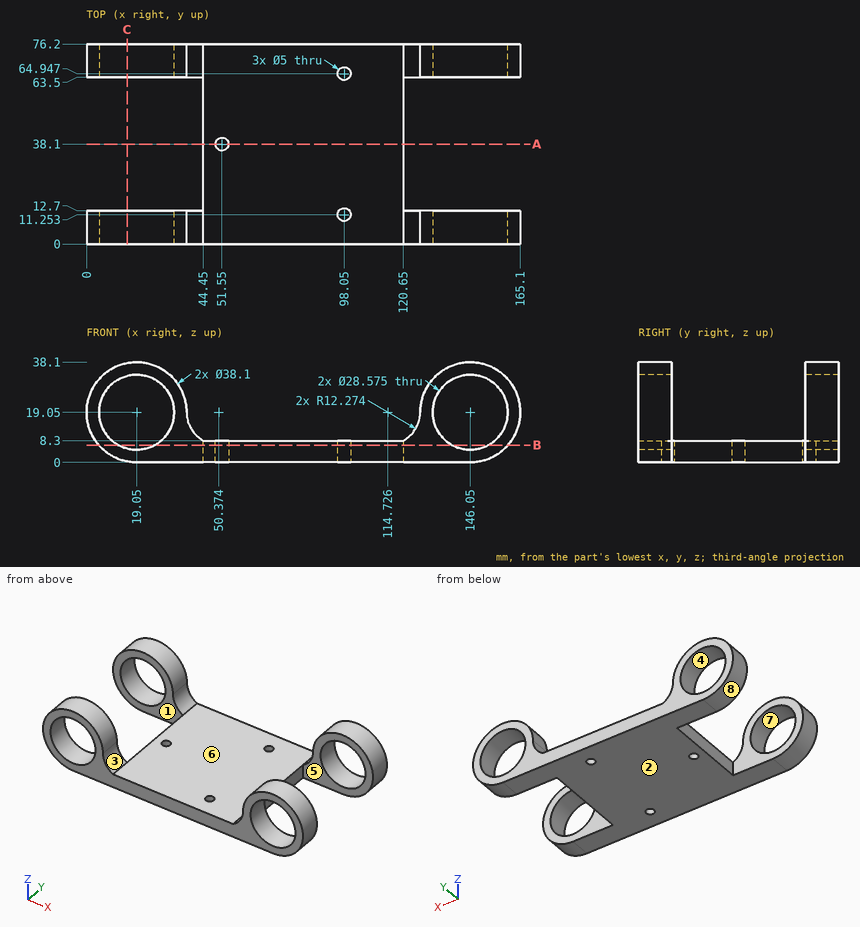
Source: three-view drawing plus pictorial views. Frame: mm from the lowest corner of the part. A direction names the side the tool comes from. Round coordinates to 2 decimals unless told otherwise and drop trailing zeros. Loops run counter-clockwise (first coordinate to the right, second up) from the corner with the lowest first, then second, coordinate; pieces in that order, holes last.
Q1. Section B-B on z = 6.5. State how many separate pieces and enclosed holes the cut face has, plus the area to 3 significant figures.
Q2. Pin query (flat end, axial travel): P1, Ø2.5, axis at y = 48, z = 6, coming from the -X side; P2, Ø8, axis at y = 65, z = 15, coming from the -X side; P3, Ø8, axis at x = 98.05, y = 64.95, coming from the +Z side. Return the tip coordinate at first contact, or that it passes through.
Q3. Section C-C on x = 15.5. Return loops of the section in (y, z), plus the area to 3 significant figures.
Q4. Material intervals for L1, parallel to X at y = 7, z = 19; L2, parallel to Y at x = 129, z = 11; L3, parallel to Z at x = 114.5, y = 55.5, sorted ascending.
Q5. Access query for the marked faces 1, 2, 3, 4 and 5. Directions: +Z, -Z, +X, -X, +Y, -Y. A direction counts if a zero-diameter tool reaches every point of the face in a straight line with its end or side. Return the directions, or none.
Q6. Section A-A on y = 38.1. Return loops of the section in (x, z), plus the area to 3 significant figures.
Q7. Pull-direction query (Z, two-part tool) for the marked faces 6, 7 and 8; classes: released by +Z, released by -Z, zero draft, split by the parting line, or undercut.
Evaluation:
1. separate pieces: 5
1. enclosed holes: 3
1. area: 7,070 mm2
2. P1: stops at x = 44.45
2. P2: stops at x = 0
2. P3: stops at z = 8.3
3. outline: (0, 0.33) - (12.7, 0.33) - (12.7, 5.21) - (0, 5.21) - close; (0, 32.89) - (12.7, 32.89) - (12.7, 37.77) - (0, 37.77) - close; (63.5, 0.33) - (76.2, 0.33) - (76.2, 5.21) - (63.5, 5.21) - close; (63.5, 32.89) - (76.2, 32.89) - (76.2, 37.77) - (63.5, 37.77) - close
3. area: 248 mm2
4. L1: x = 0 to 4.76, 33.34 to 38.1, 127 to 131.76, 160.34 to 165.1
4. L2: y = 0 to 12.7, 63.5 to 76.2
4. L3: z = 0 to 8.3
5. face 1: +Z, -Z, -X
5. face 2: -Z, +X, -X, +Y, -Y
5. face 3: +Z, +Y, -Y
5. face 4: +Y, -Y
5. face 5: +Z, -Z, +X
6. outline: (44.45, 0) - (49.05, 0) - (49.05, 8.3) - (44.45, 8.3) - close; (54.05, 0) - (120.65, 0) - (120.65, 8.3) - (54.05, 8.3) - close
6. area: 591 mm2
7. face 6: released by +Z
7. face 7: undercut
7. face 8: split by the parting line
